Input: part model. Units: mm. Frame: model coordinates. Coordinates: 2 decimals unless noted, no trailing zeros. Order: outer loops, then holes, each group sorted by start corner. A loop starts at its lowest first (then second) coordinate and runs counter-clockwise, first axis right, second up.
from build123d import *

# Parameters (mm, degrees)
CUT_EXTRUDE2_DEPTH = 0.254


with BuildPart() as part:
    # Sketch1 → Revolve1 (revolve)
    with BuildSketch(Plane.XY, mode=Mode.PRIVATE) as revolve1_sk:
        Polygon((0, 0), (0, 2.8575), (1.7018, 1.984375), (22.817280365, 1.984375), (25.4, 0), align=None)
    revolve(revolve1_sk.sketch.rotate(Axis((25.4, 0, 0), (-1, 0, 0)), 90), axis=Axis((25.4, 0, 0), (-1, 0, 0)))

    # Sketch2 → Cut-Extrude2 (cut)
    with BuildSketch(Plane(origin=(0, 0, 0), x_dir=(0, 0, -1), z_dir=(1, 0, 0))):
        with BuildLine():
            Line((1.787373723, 0.564567778), (0.680541301, 0.564567778))
            ThreePointArc((0.680541301, 0.564567778), (0.500936179, 0.638962656), (0.426541301, 0.818567778))
            Line((0.426541301, 0.818567778), (0.426541301, 1.824996112))
            ThreePointArc((0.426541301, 1.824996112), (0.352146424, 2.004601234), (0.172541301, 2.078996112))
            Line((0.172541301, 2.078996112), (-0.147792428, 2.078996112))
            ThreePointArc((-0.147792428, 2.078996112), (-0.327397551, 2.004601234), (-0.401792428, 1.824996112))
            Line((-0.401792428, 1.824996112), (-0.401792428, 0.818567778))
            ThreePointArc((-0.401792428, 0.818567778), (-0.476187306, 0.638962656), (-0.655792428, 0.564567778))
            Line((-0.655792428, 0.564567778), (-1.929964998, 0.564567778))
            ThreePointArc((-1.929964998, 0.564567778), (-2.10957012, 0.490172901), (-2.183964998, 0.310567778))
            Line((-2.183964998, 0.310567778), (-2.183964998, -0.002294215))
            ThreePointArc((-2.183964998, -0.002294215), (-2.10957012, -0.181899337), (-1.929964998, -0.256294215))
            Line((-1.929964998, -0.256294215), (-0.655792428, -0.256294215))
            ThreePointArc((-0.655792428, -0.256294215), (-0.476187306, -0.330689092), (-0.401792428, -0.510294215))
            Line((-0.401792428, -0.510294215), (-0.401792428, -1.900709616))
            ThreePointArc((-0.401792428, -1.900709616), (-0.327397551, -2.080314739), (-0.147792428, -2.154709616))
            Line((-0.147792428, -2.154709616), (0.256211375, -2.154709616))
            ThreePointArc((0.256211375, -2.154709616), (0.435816497, -2.080314739), (0.510211375, -1.900709616))
            Line((0.510211375, -1.900709616), (0.510211375, -0.526132959))
            ThreePointArc((0.510211375, -0.526132959), (0.584606253, -0.346527836), (0.764211375, -0.272132959))
            Line((0.764211375, -0.272132959), (1.787373723, -0.272132959))
            ThreePointArc((1.787373723, -0.272132959), (1.966978846, -0.197738081), (2.041373723, -0.018132959))
            Line((2.041373723, -0.018132959), (2.041373723, 0.310567778))
            ThreePointArc((2.041373723, 0.310567778), (1.966978846, 0.490172901), (1.787373723, 0.564567778))
        make_face()
    extrude(amount=CUT_EXTRUDE2_DEPTH, mode=Mode.SUBTRACT)


solid = part.part
Item 1: Cut plane A-A on x = 7.25. Return loops of the section in (y, z).
Response values:
outline: circle Ø3.97 at (0, 0)
Item 2: Draft query along Z for faces 1 (the face through (0, 1, 1)), 2 (the face through (0.254, 0, 0)), 3 (the face through (24.701, 0.525, 0.116)). Return one class per face: pulls with the +Z half, pulls with the -Z half, needs draft (parallel to the pull), parting line crosses it, or undercut.
Response values:
face 1: needs draft
face 2: undercut
face 3: parting line crosses it
Item 3: Cut plane B-B on x = 23.25. Return loops of the section in (y, z), then the cut area to 3 significant figures.
Response values:
outline: circle Ø3.3 at (0, 0)
area: 8.57 mm2
Item 4: Pin query (flat end, axial travel): pin 1 Ø2 at (x, z) = (6, -0.5) entering from -Y; pin 2 Ø2 at (x, y) = (8.5, -1) entering from +Z; pin 3 Ø2 at (x, y) = (20, 2) entering from +Z. Return the tip coordinate at first contact, or that it passes through.
Response values:
pin 1: stops at y = -1.98
pin 2: stops at z = 1.98
pin 3: stops at z = 1.71
Item 5: Ray query, probe 1 along X at (y, z) = (-2.5, 0.3); probe 2 along X at (y, z) = (-0.85, -2); probe 3 along Z at (x, y) = (5.5, 0.5). Return the intervals inside material, ascending.
Response values:
probe 1: x = 0 to 0.66
probe 2: x = 0 to 1.33
probe 3: z = -1.92 to 1.92
